```python
from build123d import *

# Parameters (mm, degrees)
SKETCH_W        = 49
SKETCH_H        = 20.5
PAD_DEPTH       = 4
POCKET_DEPTH    = 2
SKETCH002_W     = 23.5
SKETCH002_H     = 17.5
POCKET001_DEPTH = 2
SKETCH004_W     = 1
SKETCH004_H     = 14
POCKET002_DEPTH = 2
SKETCH005_W     = 1.5
SKETCH005_H     = 14
PAD001_DEPTH    = 14


with BuildPart() as part:
    # Sketch → Pad (new body)
    with BuildSketch(Plane.XY):
        with Locations((24.5, 10.25)):
            Rectangle(SKETCH_W, SKETCH_H)
    extrude(amount=PAD_DEPTH)

    # Sketch001 (on Face6 of Pad) → Pocket (cut)
    with BuildSketch(Plane.XY.offset(4)):
        Polygon((1.5, 19), (22.5, 19), (22.5, 1.5), (1.5, 1.5), (1.5, 4.5), (0, 4.5), (0, 16), (1.5, 16), align=None)
    extrude(amount=-POCKET_DEPTH, mode=Mode.SUBTRACT)

    # Sketch002 (on Face5 of Pocket) → Pocket001 (cut)
    with BuildSketch(Plane.XY.offset(4)):
        with Locations((35.75, 10.25)):
            Rectangle(SKETCH002_W, SKETCH002_H)
    extrude(amount=-POCKET001_DEPTH, mode=Mode.SUBTRACT)

    # Sketch004 (on Face19 of Pocket001) → Pocket002 (cut)
    with BuildSketch(Plane.XY.offset(2)):
        with Locations((29.5, 10.25)):
            Rectangle(SKETCH004_W, SKETCH004_H)
        with Locations((42, 10.25)):
            Rectangle(SKETCH004_W, SKETCH004_H)
    extrude(amount=-POCKET002_DEPTH, mode=Mode.SUBTRACT)

    # Sketch005 (on Face27 of Pocket002) → Pad001 (join)
    with BuildSketch(Plane.XY.offset(2)):
        with Locations((40.75, 10.25)):
            Rectangle(SKETCH005_W, SKETCH005_H)
    extrude(amount=PAD001_DEPTH)


solid = part.part
```
The model under review builds one solid part; all positions refer to its coordinate system, in mm. A direction names the side the tool comes from. Round coordinates to 2 decimals unless told otherwise and drop trailing zeros. Order: outer loops, then holes, each group sorted by start corner. A loop starts at its lowest first (then second) coordinate and runs counter-clockwise, first axis right, second up. Notation, with made-up numbers: (66.5, 23.5) -> (113.5, 23.5) arc R28 ccw to (113.5, 52.5) -> close; hole circle Ø9 at (41.25, -35.5). An arc over 180 degrees is marked (long way). Use a Markdown table: item, result.
Q1. Clearance check with flat-ended pins moving along their axes: P1, Ø6, axis at x = 21.5, y = 9, coming from the +Z side; P2, Ø4, axis at y = 7, z = 6.5, coming from the -X side; P3, Ø4, axis at y = 2, z = 11, coming from the +X side. State where each tip first meets the part, or that it passes through.
Values:
| item | result |
|---|---|
| P1 | stops at z = 4 |
| P2 | stops at x = 40 |
| P3 | stops at x = 41.5 |
Q2. For line 1 (X direction, y = 5, z = 3); line 2 (X direction, y = 2.75, z = 2.25); line 3 (Z direction, x = 13, y = 2), list the stretches that pass through material, from the lowest coordinate up.
Values:
| item | result |
|---|---|
| line 1 | x = 22.5 to 24, 40 to 41.5, 47.5 to 49 |
| line 2 | x = 0 to 1.5, 22.5 to 24, 47.5 to 49 |
| line 3 | z = 0 to 2 |
Q3. We need section D-D on z = 11.75. Write out the cut boundary in (x, y), then the cut area to 3 significant figures.
Values:
| item | result |
|---|---|
| outline | (40, 3.25) -> (41.5, 3.25) -> (41.5, 17.25) -> (40, 17.25) -> close |
| area | 21.0 mm^2 |
Q4. We need section B-B on x = 41. Write out the cut boundary in (y, z).
Values:
| item | result |
|---|---|
| outline | (0, 0) -> (20.5, 0) -> (20.5, 4) -> (19, 4) -> (19, 2) -> (17.25, 2) -> (17.25, 16) -> (3.25, 16) -> (3.25, 2) -> (1.5, 2) -> (1.5, 4) -> (0, 4) -> close |
Q5. We need section A-A on y = 14.5. Write out the cut boundary in (x, z).
Values:
| item | result |
|---|---|
| outline | (0, 0) -> (29, 0) -> (29, 2) -> (24, 2) -> (24, 4) -> (22.5, 4) -> (22.5, 2) -> (0, 2) -> close; (30, 0) -> (41.5, 0) -> (41.5, 16) -> (40, 16) -> (40, 2) -> (30, 2) -> close; (42.5, 0) -> (49, 0) -> (49, 4) -> (47.5, 4) -> (47.5, 2) -> (42.5, 2) -> close |
Q6. We need section C-C on y = 2.5. Write out the cut boundary in (x, z), then the cut area to 3 significant figures.
Values:
| item | result |
|---|---|
| outline | (0, 0) -> (49, 0) -> (49, 4) -> (47.5, 4) -> (47.5, 2) -> (24, 2) -> (24, 4) -> (22.5, 4) -> (22.5, 2) -> (1.5, 2) -> (1.5, 4) -> (0, 4) -> close |
| area | 107 mm^2 |
Q7. Mouldability with a two-part tool opening along Y and no side actions: class faces 1 (the flat face through (1, 16, 3)), 2 (the flat face through (0, 10.1, 1.5)) as +Y half, -Y half, draft (parallel to the pull), parting line (faces both ways), or undercut.
Values:
| item | result |
|---|---|
| face 1 | undercut |
| face 2 | draft |
Q8. Tool access review of faces 3 (the flat face through (49, 10, 2)), 4 (the flat face through (1, 4.5, 3)), 5 (the flat face through (29, 10, 1)), 6 (the flat face through (24, 10, 0)), 7 (the flat face through (36, 19, 3)): name each direction out of +Z, -Z, +X, -X, +Y, -Y from which nothing blocks a thin tool from reaching the whole face with its end or side.
Values:
| item | result |
|---|---|
| face 3 | +Z, -Z, +X, +Y, -Y |
| face 4 | +Z, -X |
| face 5 | +Z, -Z |
| face 6 | -Z, +X, -X, +Y, -Y |
| face 7 | +Z |
